Autodesk Inventor part; units mm, degrees
ref_plane "Work Plane1" through (-15, 0, 0) normal (-1, 0, 0) x (0, 0, 1)
ref_plane "YZ Plane" through (0, 0, 0) normal (1, 0, 0) x (0, 1, 0)
ref_plane "XZ Plane" through (0, 0, 0) normal (0, 1, 0) x (-1, 0, 0)
sketch "Sketch1" plane through (0, 0, 0) normal (0, 1, 0) x (-1, 0, 0)
  circle A0 centre (0, 0) radius 15
  line L0 (0, -15) -> (0, 15)
  dimension "d0" = 30
extrude "Extrusion2" add sketch "Sketch1" along normal mid plane 11.5 contours A0 L0 picked at (3.1174, 3.9092)
sketch "Sketch2" plane through (0, 5.75, 0) normal (0, 1, 0) x (1, 0, 0)
  line L0 (0, -15) -> (0, 15)
  line L1 (0, -15) -> (-17, -15)
  line L2 (-17, -15) -> (-17, 15)
  line L3 (-17, 15) -> (0, 15)
  line L4 (0, 15) -> (0, -15)
  point P0 (0, 0)
extrude "Extrusion3" add sketch "Sketch2" against normal blind 2
sketch "Sketch3" plane through (0, -5.75, 0) normal (0, -1, 0) x (1, 0, 0)
  arc A0 (0, 15) -> (0, -15) centre (0, 0) ccw
  line L0 (-17, 15) -> (-17, -15)
  line L1 (0, -15) -> (-17, -15)
  line L2 (-17, -15) -> (-17, 15)
  line L3 (-17, 15) -> (0, 15)
  line L4 (0, 15) -> (0, -15)
extrude "Extrusion4" add sketch "Sketch3" against normal blind 2 contours A0 L1 L0 L3
ref_plane "Work Plane1" through (-15, 0, 0) normal (-1, 0, 0) x (0, 0, 1)
sketch "Sketch5" plane through (-15, 0, 0) normal (-1, 0, 0) x (0, 0, 1)
  circle A0 centre (-5, 0) radius 1.6
  line L0 (-15, 3.75) -> (-15, -3.75)
  circle A1 centre (5, 0) radius 1.6
  line L1 (15, -3.75) -> (15, 3.75)
  circle A2 centre (-5, 0) radius 2.75
  circle A3 centre (5, 0) radius 2.75
  point P0 (0, 0)
  dimension "d10" = 3.2
  dimension "d11" = 10
  dimension "d12" = 3.2
  dimension "d13" = 10
  dimension "d14" = 5.5
  dimension "d15" = 5.5
extrude "Extrusion5" cut sketch "Sketch5" against normal blind 15 contours A0 | A1
extrude "Extrusion6" cut sketch "Sketch5" against normal blind 9
fillet "Fillet1" radius 5 4 edges at (-17, 4.75, -15) (-17, 4.75, 15) (-17, -4.75, 15) (-17, -4.75, -15)
properties part number "Katrol Lifter_3DPrint"
Read the model definition and answer for the solid it produces. Units are mm, in the model's axes. A direction names the side the tool comes from. Coordinates: 2 decimals unless noted, no trailing zeros. Loops run counter-clockwise (first coordinate to the right, second up) from the corner with the lowest first, then second, coordinate; pieces in that order, holes last. Notation, with made-up numbers: (-9.75, 46) -> (19.25, 46) arc R7 ccw to (19.25, 56) -> close; hole circle Ø9 at (-11, 23). An arc over 180 degrees is marked (long way). Write item = value, one per line. Start each with the question number.
1) The part is cut by section C-C, the plane x = -11. Determine the outline of the cut face in (y, z).
2) The part is cut by section D-D, the plane z = -9. Determine the outline of the cut face in (x, y).
3) The part is cut by section A-A, the plane z = -5. Determine the outline of the cut face in (x, y), plus the area to 3 significant figures.
4) For faces 1 (the face through (-15, -5, -14)), 2 (the face through (-15.5, -3.75, -1)), determine the directions among +Z, -Z, +X, -X, +Y, -Y from which every point of the face is accessible in a straight line to the end or side of a thin tool.
5) The part is cut by section B-B, the plane y = 0.5. Determine the outline of the cut face in (x, z), plus the area to 3 significant figures.
6) The mould has two halves that part along Z. Classify faces 3 (the face through (-6, 5, 15)), 4 (the face through (-6, 0, 7)), 5 (the face through (-17, -5, 0)), 6 (the face through (-3.04, 0.07, 3.4)): pulls with the +Z half, pulls with the -Z half, needs draft (parallel to the pull), parting line crosses it, or undercut.
7) Find the intervals of material crossed by L1, parallel to Y at x = -4.7, z = 5; L2, parallel to Z at x = -9.25, y = -2.25; L3, parallel to Y at x = -9, z = -5, in increasing order. Write a range as from..to.
8) Given P1, Ø4, axis at y = 0, z = 5, coming from the +X side; P2, Ø2, axis at x = -13, y = 0.5, coming from the -Z side; P3, Ø1, axis at x = -14, y = -0.5, coming from the +Z side; P4, Ø3, axis at y = 0, z = 4, coming from the -X side, each flat-ended and moving along its own axis, determine where each tip first touches the part or whether it passes through.
Result:
q1.outline = (-5.75, -15) -> (-3.75, -15) -> (-3.75, -10.2) -> (3.75, -10.2) -> (3.75, -15) -> (5.75, -15) -> (5.75, 15) -> (3.75, 15) -> (3.75, 10.2) -> (-3.75, 10.2) -> (-3.75, 15) -> (-5.75, 15) -> close; hole circle Ø5.5 at (0, -5); hole circle Ø5.5 at (0, 5)
q2.outline = (-17, -5.75) -> (0, -5.75) -> (0, 5.75) -> (-17, 5.75) -> (-17, 3.75) -> (-12, 3.75) -> (-12, -3.75) -> (-17, -3.75) -> close
q3.outline = (-17, -5.75) -> (0, -5.75) -> (0, -1.6) -> (-6, -1.6) -> (-6, -2.75) -> (-14.14, -2.75) -> (-14.14, -3.75) -> (-17, -3.75) -> close; (-17, 3.75) -> (-14.14, 3.75) -> (-14.14, 2.75) -> (-6, 2.75) -> (-6, 1.6) -> (0, 1.6) -> (0, 5.75) -> (-17, 5.75) -> close
q3.area = 110 mm²
q4.face_1 = -Z, -X, +Y, -Y
q4.face_2 = -X
q5.outline = (-14.82, -2.3) -> (-6, -2.3) -> (-6, -3.48) -> (0, -3.48) -> (0, 3.48) -> (-6, 3.48) -> (-6, 2.3) -> (-14.82, 2.3) arc R15 ccw to start; (-12.87, -7.7) arc R15 ccw to (0, -15) -> (0, -6.52) -> (-6, -6.52) -> (-6, -7.7) -> close; (-12.87, 7.7) -> (-6, 7.7) -> (-6, 6.52) -> (0, 6.52) -> (0, 15) arc R15 ccw to start
q5.area = 230 mm²
q6.face_3 = pulls with the +Z half
q6.face_4 = undercut
q6.face_5 = needs draft
q6.face_6 = undercut
q7.L1 = -5.75..-1.6, 1.6..5.75
q7.L2 = -11.81..-6.58, -3.42..3.42, 6.58..11.81
q7.L3 = -5.75..-2.75, 2.75..5.75
q8.P1 = 0
q8.P2 = -9
q8.P3 = 2.44
q8.P4 = -6
